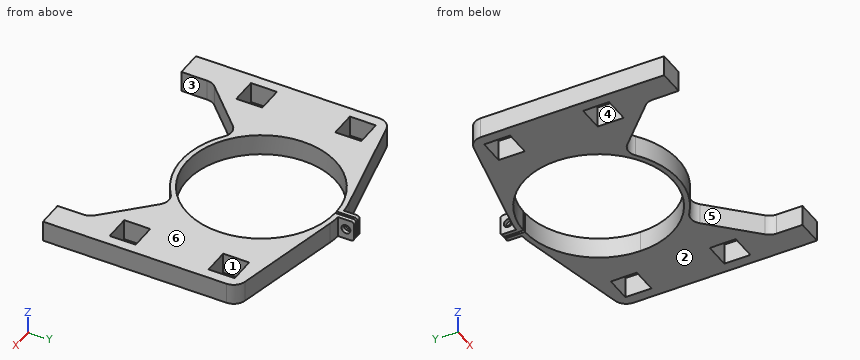
```python
from build123d import *

# Parameters (mm, degrees)
SKIZZE1_R                       = 30.65
SKIZZE1_R_2                     = 28.65
AUFSATZ_LINEAR_AUSTRAGEN1_DEPTH = 8
AUFSATZ_LINEAR_AUSTRAGEN2_DEPTH = 8
SKIZZE3_W                       = 1
SKIZZE3_H                       = 2.855309686
SCHNITT_LINEAR_AUSTRAGEN1_DEPTH = 10
AUFSATZ_LINEAR_AUSTRAGEN3_DEPTH = 8
SKIZZE5_R                       = 1.7
SCHNITT_LINEAR_AUSTRAGEN2_DEPTH = 8
VERRUNDUNG2_R                   = 1
SKIZZE7_W                       = 10
SKIZZE7_H                       = 10
SCHNITT_LINEAR_AUSTRAGEN4_DEPTH = 10
VERRUNDUNG3_R                   = 5


with BuildPart() as part:
    # Skizze1 → Aufsatz-Linear austragen1 (new body)
    with BuildSketch(Plane.XY):
        Circle(SKIZZE1_R)
        Circle(SKIZZE1_R_2, mode=Mode.SUBTRACT)
    extrude(amount=AUFSATZ_LINEAR_AUSTRAGEN1_DEPTH)

    # Skizze2 → Aufsatz-Linear austragen2 (add)
    with BuildSketch(Plane.XY.offset(8)):
        with BuildLine():
            Line((42.5, -42.5), (42.5, -54.5))
            Line((42.5, -54.5), (52.5, -54.5))
            Line((52.5, -54.5), (52.5, 20))
            Line((52.5, 20), (6.481641536, 29.956815969))
            Line((6.481641536, 29.956815969), (6.460494255, 29.859077581))
            ThreePointArc((6.460494255, 29.859077581), (29.307694933, 8.623312455), (21.602112165, -21.602112165))
            Line((21.602112165, -21.602112165), (21.672822843, -21.672822843))
            Line((21.672822843, -21.672822843), (42.5, -42.5))
        make_face()
        with BuildLine():
            Line((-21.672822843, -21.672822843), (-42.5, -42.5))
            Line((-42.5, -42.5), (-42.5, -54.5))
            Line((-42.5, -54.5), (-52.5, -54.5))
            Line((-52.5, -54.5), (-52.5, 20))
            Line((-52.5, 20), (-6.481641536, 29.956815969))
            Line((-6.481641536, 29.956815969), (-6.460494255, 29.859077581))
            ThreePointArc((-6.460494255, 29.859077581), (-29.307694933, 8.623312455), (-21.602112165, -21.602112165))
            Line((-21.602112165, -21.602112165), (-21.672822843, -21.672822843))
        make_face()
    extrude(amount=-AUFSATZ_LINEAR_AUSTRAGEN2_DEPTH)

    # Skizze3 → Schnitt-Linear austragen1 (cut)
    with BuildSketch(Plane.XY.offset(8)):
        with Locations((0, 29.34103969)):
            Rectangle(SKIZZE3_W, SKIZZE3_H)
    extrude(amount=-SCHNITT_LINEAR_AUSTRAGEN1_DEPTH, mode=Mode.SUBTRACT)

    # Skizze4 → Aufsatz-Linear austragen3 (add)
    with BuildSketch(Plane.XY.offset(8)):
        Polygon((0.5, 30.645921425), (0.5, 36.645921425), (2, 36.645921425), (2, 29.02715443), align=None)
        Polygon((-2, 29.02715443), (-0.5, 30.645921425), (-0.5, 36.645921425), (-2, 36.645921425), align=None)
    extrude(amount=-AUFSATZ_LINEAR_AUSTRAGEN3_DEPTH)

    # Skizze5 → Schnitt-Linear austragen2 (cut)
    with BuildSketch(Plane.ZY.offset(2)):
        with Locations(Location((4, 33.615299481, 0), (0, 0, 270))):
            Circle(SKIZZE5_R)
    extrude(amount=-SCHNITT_LINEAR_AUSTRAGEN2_DEPTH, mode=Mode.SUBTRACT)

    # Verrundung2
    verrundung2_edges = [part.edges().sort_by_distance(p)[0] for p in [
        (-1.25, 36.645921425, 8),
        (-1.25, 36.645921425, 0),
        (1.25, 36.645921425, 8),
        (1.25, 36.645921425, 0),
    ]]
    fillet(verrundung2_edges, radius=VERRUNDUNG2_R)

    # Skizze7 → Schnitt-Linear austragen4 (cut)
    with BuildSketch(Plane(origin=(0, 0, 0), x_dir=(-1, 0, 0), z_dir=(0, 0, -1))):
        with Locations((-43.5, 11.86546468)):
            Rectangle(SKIZZE7_W, SKIZZE7_H)
        with Locations((-43.5, -26.13453532)):
            Rectangle(SKIZZE7_W, SKIZZE7_H)
        with Locations((43.5, -26.13453532)):
            Rectangle(SKIZZE7_W, SKIZZE7_H)
        with Locations((43.5, 11.86546468)):
            Rectangle(SKIZZE7_W, SKIZZE7_H)
    extrude(amount=-SCHNITT_LINEAR_AUSTRAGEN4_DEPTH, mode=Mode.SUBTRACT)

    # Verrundung3
    verrundung3_edges = [part.edges().sort_by_distance(p)[0] for p in [
        (-21.672822843, -21.672822843, 4),
        (-42.5, -42.5, 4),
        (-52.5, 20, 4),
        (21.672822843, -21.672822843, 4),
        (42.5, -42.5, 4),
        (52.5, 20, 4),
    ]]
    fillet(verrundung3_edges, radius=VERRUNDUNG3_R)


solid = part.part
```
Check sheet for the modelled part. Datum: model origin and axes. Units: mm. Face numbers are marked on the shaded views. A direction names the side the tool comes from. Round coordinates to 2 decimals unless told otherwise and drop trailing zeros. Write each loop counter-clockwise with the first axis right and the second up, starting at its lowest first coordinate (ties: lowest second). Pieces come first, ordered by that corner, then holes. Notation, with made-up numbers: (8.25, 33) -> (41.25, 33) arc R24 cw to (41.25, 66) -> close; hole circle Ø11 at (12, -24). An arc over 180 degrees is marked (long way). Put each result on its own line as item: value.
(1) Go/stop test with flat-tipped pins: pin 1 Ø3 at (x, z) = (5, 2) entering from +Y; pin 2 Ø2.5 at (y, z) = (33, 2.5) entering from -X; pin 3 Ø1 at (x, z) = (13, 3.5) entering from +Y. Record where each tip stops, or that it passes through.
Values found:
pin 1: stops at y = 30.45
pin 2: stops at x = -2
pin 3: stops at y = 28.65
(2) Material ranges on line 1 (X direction, y = -22, z = 2); line 2 (X direction, y = 0, z = 3.5); line 3 (X direction, y = 15.5, z = 7), recorded low to high.
Values found:
line 1: x = -52.5 to -48.5, -38.5 to -18.35, 18.35 to 38.5, 48.5 to 52.5
line 2: x = -52.5 to -28.65, 28.65 to 52.5
line 3: x = -52.5 to -48.5, -38.5 to -24.1, 24.1 to 38.5, 48.5 to 52.5
(3) Sectioned sample at C-C (z = 4). Count the separate pieces of the cut face and the enclosed holes in it, plus the area to 3 significant figures.
Values found:
separate pieces: 3
enclosed holes: 4
area: 3,360 mm^2
(4) Mould release check, pull along Y, two halves, no side actions. Record for the marked faces 4, 5 and 6: released by +Y, released by -Y, zero draft, split by the parting line, or undercut.
Values found:
face 4: undercut
face 5: released by -Y
face 6: zero draft
(5) Sectioned sample at D-D (y = -27.5). Enter the section's corners in (x, z), plus the area to 3 significant figures.
Values found:
outline: (-52.5, 0) -> (-48.5, 0) -> (-48.5, 8) -> (-52.5, 8) -> close; (-38.5, 0) -> (-27.5, 0) -> (-27.5, 8) -> (-38.5, 8) -> close; (-13.53, 0) -> (-8.04, 0) -> (-8.04, 8) -> (-13.53, 8) -> close; (8.04, 0) -> (13.53, 0) -> (13.53, 8) -> (8.04, 8) -> close; (27.5, 0) -> (38.5, 0) -> (38.5, 8) -> (27.5, 8) -> close; (48.5, 0) -> (52.5, 0) -> (52.5, 8) -> (48.5, 8) -> close
area: 328 mm^2
(6) Tool access check on the marked faces 1, 2 and 3. Record the directions out of +Z, -Z, +X, -X, +Y, -Y that give a thin tool (end or side, any length) a straight path to the whole face; none if there is none.
Values found:
face 1: +Z, -Z
face 2: -Z, +X, -X, +Y, -Y
face 3: +Z, -Z, -Y
(7) Sectioned sample at B-B (x = 20.5). Enter the section's corners in (y, z).
Values found:
outline: (-23.58, 0) -> (-20.01, 0) -> (-20.01, 8) -> (-23.58, 8) -> close; (20.01, 0) -> (26.92, 0) -> (26.92, 8) -> (20.01, 8) -> close
(8) Sectioned sample at A-A (y = -8). Enter the section's corners in (x, z).
Values found:
outline: (-52.5, 0) -> (-27.51, 0) -> (-27.51, 8) -> (-52.5, 8) -> close; (27.51, 0) -> (52.5, 0) -> (52.5, 8) -> (27.51, 8) -> close
